Input: part model. Units: mm. Frame: model coordinates. A direction names the side the tool comes from. Give positions to 0.01 mm unless a question says otherwise; leave off trailing zeros. Loops run counter-clockwise (first coordinate to the right, second up) from the corner with the lowest first, then second, coordinate; pieces in that order, holes last. Notation, with made-up numbers: M 30,63 L 39,63 A23 cw 39,102 Z; hole C 39,-22 d4. An arc over 180 degrees is marked long. Use a Markdown table: item, result. Add a question column.
from build123d import *

# Parameters (mm, degrees)
BOSS_EXTRUDE1_DEPTH = 8
SKETCH2_R           = 8
BOSS_EXTRUDE2_DEPTH = 1.3
BOSS_EXTRUDE3_START = 7.5
SKETCH3_R           = 8
BOSS_EXTRUDE3_DEPTH = 7.5
SKETCH4_R           = 2.5
CUT_EXTRUDE1_DEPTH  = 18.5
SKETCH5_R           = 1.5
CUT_EXTRUDE2_DEPTH  = 10.5
SKETCH6_R           = 1.5
CUT_EXTRUDE3_DEPTH  = 16.5


with BuildPart() as part:
    # Sketch1 → Boss-Extrude1 (new body)
    with BuildSketch(Plane(origin=(0, 0, 0), x_dir=(1, 0, 0), z_dir=(0, 1, 0))):
        with BuildLine():
            ThreePointArc((-2.435695647, 5.042557557), (-2.542346799, 4.989636535), (-2.647848779, 4.934460137))
            ThreePointArc((-2.647848779, 4.934460137), (-2.844880621, 3.915642253), (-3.874720197, 4.043085876))
            ThreePointArc((-3.874720197, 4.043085876), (-3.959797975, 3.959797975), (-4.043085876, 3.874720197))
            ThreePointArc((-4.043085876, 3.874720197), (-3.915642253, 2.844880621), (-4.934460137, 2.647848779))
            ThreePointArc((-4.934460137, 2.647848779), (-4.989636535, 2.542346799), (-5.042557557, 2.435695647))
            ThreePointArc((-5.042557557, 2.435695647), (-4.603113539, 1.495642253), (-5.511180739, 0.993421795))
            ThreePointArc((-5.511180739, 0.993421795), (-5.531054707, 0.876033004), (-5.548428571, 0.758248236))
            ThreePointArc((-5.548428571, 0.758248236), (-4.84, 0), (-5.548428571, -0.758248236))
            ThreePointArc((-5.548428571, -0.758248236), (-5.531054707, -0.876033004), (-5.511180739, -0.993421795))
            ThreePointArc((-5.511180739, -0.993421795), (-4.603113539, -1.495642253), (-5.042557557, -2.435695647))
            ThreePointArc((-5.042557557, -2.435695647), (-4.989636535, -2.542346799), (-4.934460137, -2.647848779))
            ThreePointArc((-4.934460137, -2.647848779), (-3.915642253, -2.844880621), (-4.043085876, -3.874720197))
            ThreePointArc((-4.043085876, -3.874720197), (-3.959797975, -3.959797975), (-3.874720197, -4.043085876))
            ThreePointArc((-3.874720197, -4.043085876), (-2.844880621, -3.915642253), (-2.647848779, -4.934460137))
            ThreePointArc((-2.647848779, -4.934460137), (-2.542346799, -4.989636535), (-2.435695647, -5.042557557))
            ThreePointArc((-2.435695647, -5.042557557), (-1.495642253, -4.603113539), (-0.993421795, -5.511180739))
            ThreePointArc((-0.993421795, -5.511180739), (-0.876033004, -5.531054707), (-0.758248236, -5.548428571))
            ThreePointArc((-0.758248236, -5.548428571), (0, -4.84), (0.758248236, -5.548428571))
            ThreePointArc((0.758248236, -5.548428571), (0.876033004, -5.531054707), (0.993421795, -5.511180739))
            ThreePointArc((0.993421795, -5.511180739), (1.495642253, -4.603113539), (2.435695647, -5.042557557))
            ThreePointArc((2.435695647, -5.042557557), (2.542346799, -4.989636535), (2.647848779, -4.934460137))
            ThreePointArc((2.647848779, -4.934460137), (2.844880621, -3.915642253), (3.874720197, -4.043085876))
            ThreePointArc((3.874720197, -4.043085876), (3.959797975, -3.959797975), (4.043085876, -3.874720197))
            ThreePointArc((4.043085876, -3.874720197), (3.915642253, -2.844880621), (4.934460137, -2.647848779))
            ThreePointArc((4.934460137, -2.647848779), (4.989636535, -2.542346799), (5.042557557, -2.435695647))
            ThreePointArc((5.042557557, -2.435695647), (4.603113539, -1.495642253), (5.511180739, -0.993421795))
            ThreePointArc((5.511180739, -0.993421795), (5.531054707, -0.876033004), (5.548428571, -0.758248236))
            ThreePointArc((5.548428571, -0.758248236), (4.84, 0), (5.548428571, 0.758248236))
            ThreePointArc((5.548428571, 0.758248236), (5.531054707, 0.876033004), (5.511180739, 0.993421795))
            ThreePointArc((5.511180739, 0.993421795), (4.603113539, 1.495642253), (5.042557557, 2.435695647))
            ThreePointArc((5.042557557, 2.435695647), (4.989636535, 2.542346799), (4.934460137, 2.647848779))
            ThreePointArc((4.934460137, 2.647848779), (3.915642253, 2.844880621), (4.043085876, 3.874720197))
            ThreePointArc((4.043085876, 3.874720197), (3.959797975, 3.959797975), (3.874720197, 4.043085876))
            ThreePointArc((3.874720197, 4.043085876), (2.844880621, 3.915642253), (2.647848779, 4.934460137))
            ThreePointArc((2.647848779, 4.934460137), (2.542346799, 4.989636535), (2.435695647, 5.042557557))
            ThreePointArc((2.435695647, 5.042557557), (1.495642253, 4.603113539), (0.993421795, 5.511180739))
            ThreePointArc((0.993421795, 5.511180739), (0.876033004, 5.531054707), (0.758248236, 5.548428571))
            ThreePointArc((0.758248236, 5.548428571), (0, 4.84), (-0.758248236, 5.548428571))
            ThreePointArc((-0.758248236, 5.548428571), (-0.876033004, 5.531054707), (-0.993421795, 5.511180739))
            ThreePointArc((-0.993421795, 5.511180739), (-1.495642253, 4.603113539), (-2.435695647, 5.042557557))
        make_face()
    extrude(amount=BOSS_EXTRUDE1_DEPTH)

    # Sketch2 → Boss-Extrude2 (add)
    with BuildSketch(Plane(origin=(0, 8, 0), x_dir=(1, 0, 0), z_dir=(0, 1, 0))):
        with Locations(Location((0, 0, 0), (0, 0, 270))):
            Circle(SKETCH2_R)
    extrude(amount=BOSS_EXTRUDE2_DEPTH)

    # Sketch3 → Boss-Extrude3 (add)
    with BuildSketch(Plane.XZ.offset(BOSS_EXTRUDE3_START)):
        with Locations(Location((0, 0, 0), (0, 0, 90))):
            Circle(SKETCH3_R)
    extrude(amount=-BOSS_EXTRUDE3_DEPTH)

    # Sketch4 → Cut-Extrude1 (cut)
    with BuildSketch(Plane.XZ.offset(7.5)):
        with Locations(Location((0, 0, 0), (0, 0, 270))):
            Circle(SKETCH4_R)
    extrude(amount=-CUT_EXTRUDE1_DEPTH, mode=Mode.SUBTRACT)

    # Sketch5 → Cut-Extrude2 (cut)
    with BuildSketch(Plane(origin=(0, 0, 0), x_dir=(0, 0, -1), z_dir=(1, 0, 0))):
        with Locations(Location((0, -3.75, 0), (0, 0, 180))):
            Circle(SKETCH5_R)
    extrude(amount=CUT_EXTRUDE2_DEPTH, mode=Mode.SUBTRACT)

    # Sketch6 → Cut-Extrude3 (cut)
    with BuildSketch(Plane.XY):
        with Locations(Location((0, -3.75, 0), (0, 0, 180))):
            Circle(SKETCH6_R)
    extrude(amount=CUT_EXTRUDE3_DEPTH, mode=Mode.SUBTRACT)


solid = part.part
1) Section query A-A, the plane y = -3.75. Return the cut outline in (x, z).
2) Section query D-D, the plane y = -0.75. Return the cut outline in (x, z).
3) Contact query for flat-ended pins moving along their axis: P1, Ø3, axis at x = 5.5, y = 4, coming from the -Z side; P2, Ø5, axis at y = -2.5, z = -0.5, coming from the -X side; P3, Ø3, axis at x = -5.5, y = 3, coming from the +Z side; P4, Ø1.5, axis at x = -3, y = -5, coming from the +Z side. Output: stop coordinate, or through.
4) Reachability of faces 1 (the cylindrical face through (-3.925, 3.944, 2.832)), 2 (the cylindrical face through (7.81, -3.8, -1.73)), 3 (the cylindrical face through (-0.02, 3.94, 4.84)) from +Z, -Z, +X, -X, +Y, -Y: full face, straight path, thin tool, end or side. Return the list, or none.
5) Section query C-C, the plane x = 1.25. Return the cut outline in (y, z).
6) Pull-direction query (X, two-part tool) for faces 4 (the flat face through (-2, -7.5, 2)), 5 (the cylindrical face through (4.84, 3.94, 0.02)), 6 (the cylindrical face through (3.925, 3.944, -2.832)); classes: pulls with the +X half, pulls with the -X half, needs draft (parallel to the pull), parting line crosses it, or undercut.
7) Section query B-B, the plane z = 0. Return the cut outline in (x, y).
8) Ray query, line 1 (Y direction, x = 5, z = 0); line 2 (Y direction, x = -2, z = 6); line 3 (X direction, y = 2.75, z = 0). Return the intervals inside material, ascending. Write a range as [from, to].
Entries:
| question | item | result |
|---|---|---|
| 1 | outline | M -1.5,2 L -1.5,7.86 A8 ccw long 7.86,-1.5 L 2,-1.5 A2.5 cw long Z; M 1.5,2 A2.5 cw 2,1.5 L 7.86,1.5 A8 ccw 1.5,7.86 Z |
| 2 | outline | C 0,0 d16; hole C 0,0 d5 |
| 3 | P1 | stops at z = -3.92 |
| 3 | P2 | stops at x = -8 |
| 3 | P3 | stops at z = 3.92 |
| 3 | P4 | stops at z = 7.68 |
| 4 | face 1 | none |
| 4 | face 2 | +Y, -Y |
| 4 | face 3 | +Z |
| 5 | outline | M -7.5,-7.9 L 0,-7.9 L 0,-4.74 L 8,-4.74 L 8,-7.9 L 9.3,-7.9 L 9.3,-2.17 L -7.5,-2.17 Z; M -7.5,2.17 L -4.58,2.17 L -4.58,7.9 L -7.5,7.9 Z; M -2.92,2.17 L 9.3,2.17 L 9.3,7.9 L 8,7.9 L 8,4.74 L 0,4.74 L 0,7.9 L -2.92,7.9 Z |
| 6 | face 4 | needs draft |
| 6 | face 5 | pulls with the +X half |
| 6 | face 6 | undercut |
| 7 | outline | M -8,-7.5 L -2.5,-7.5 L -2.5,9.3 L -8,9.3 L -8,8 L -4.84,8 L -4.84,0 L -8,0 Z; M 2.5,-7.5 L 8,-7.5 L 8,-5.25 L 2.5,-5.25 Z; M 2.5,-2.25 L 8,-2.25 L 8,0 L 4.84,0 L 4.84,8 L 8,8 L 8,9.3 L 2.5,9.3 Z |
| 8 | line 1 | y = [-7.5, -5.25], [-2.25, 0], [8, 9.3] |
| 8 | line 2 | y = [-7.5, 0], [8, 9.3] |
| 8 | line 3 | x = [-4.84, -2.5], [2.5, 4.84] |
